CAD build for the part. Positions are in the model's coordinates, mm. Face numbers are marked on the shaded views. A direction names the side the tool comes from. Give positions to 0.01 mm unless a question says otherwise; leave off trailing zeros. Write each loop counter-clockwise with the first axis right and the second up, starting at its lowest first coordinate (ties: lowest second). Pieces come first, ordered by that corner, then holes. Notation, with made-up numbers: (36.25, 69) - (53.25, 69) arc R27 ccw to (53.25, 107) - close; hole circle Ø3 at (61.25, 64.25). An arc over 180 degrees is marked (long way). Put each result on its own line as item: value. Start each with the question number.
1. Cut at A-A on z = 270. List the corners of the cut face in (x, y).
2. Wall check: line 1 (Y direction, x = 126, z = 883); line 2 (Y direction, x = -24.5, z = 349); line 3 (X direction, y = 32, z = 335). Give the ranges that are in metal, low to high.
3. Drop flat-ended pins along their axis: pin 1 (9 mm diameter, centred on x = 5.5, y = -106.5, fed in from +Z); pin 2 (6 mm diameter, centred on x = 85, y = 5.5, fed in from -Z); pin 3 (1 mm diameter, centred on x = 45.5, z = 158, fed in from +Y). Give the stop position or say it passes through.
4. Cut at C-C on x = 117. List the corners of the cut face in (y, z), and give its area (3 significant figures).
5. Tool access for the marked faces 1, 2 and 3: list every direction of +Z, -Z, +X, -X, +Y, -Y with a clear straight run to the whole face (end or side of a thin tool).
6. Cut at B-B on x = 68.5. List the corners of the cut face in (y, z).
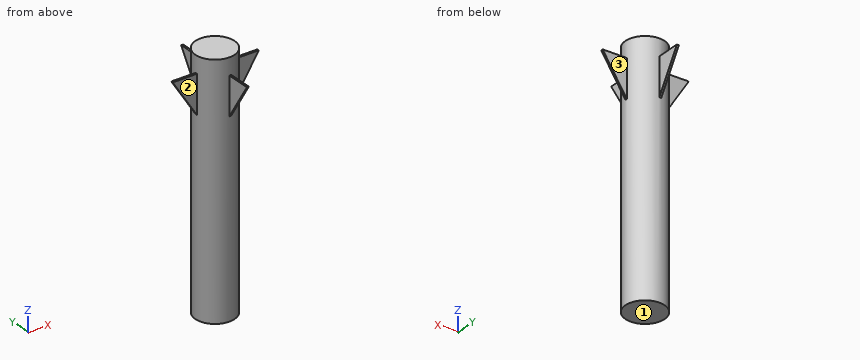
from build123d import *

# Parameters (mm, degrees)
SZKIC1_R                    = 80
DODANIE_WYCI_GNI_CIE1_DEPTH = 1000
DODANIE_WYCI_GNI_CIE2_DEPTH = 8
SZYK_KO_OWY1_COUNT          = 4


with BuildPart() as part:
    # Szkic1 → Dodanie-wyciągnięcie1 (new body)
    with BuildSketch(Plane.XY):
        Circle(SZKIC1_R)
    extrude(amount=DODANIE_WYCI_GNI_CIE1_DEPTH)

    # Szkic5 → Dodanie-wyciągnięcie2 (add)
    with BuildSketch(Plane(origin=(0, 0, 0), x_dir=(1, 0, 0), z_dir=(0, 1, 0))):
        Polygon((73.616187197, -766.737875277), (178.616187197, -931.737875277), (73.616187197, -931.737875277), align=None)
    dodanie_wyci_gni_cie2 = extrude(amount=DODANIE_WYCI_GNI_CIE2_DEPTH)

    # Szyk kołowy1: Dodanie-wyciągnięcie2 ×4 about axis
    szyk_ko_owy1_axis = Axis((0, 0, 0), (0, 0, 1))
    for i in range(1, SZYK_KO_OWY1_COUNT):
        add(dodanie_wyci_gni_cie2.rotate(szyk_ko_owy1_axis, i * 360 / SZYK_KO_OWY1_COUNT))


solid = part.part
Report:
1. outline: circle Ø160 at (0, 0)
2. line 1: y = 0 to 8
2. line 2: y = -76.16 to 76.16
2. line 3: x = -73.32 to 73.32
3. pin 1: stops at z = 931.74
3. pin 2: stops at z = 779.91
3. pin 3: stops at y = 66.14
4. outline: (0, 834.91) - (8, 834.91) - (8, 931.74) - (0, 931.74) - close
4. area: 775 mm²
5. face 1: -Z, +X, -X, +Y, -Y
5. face 2: +Z, -Z, -X, -Y
5. face 3: +Z, -Z, +X, +Y
6. outline: (-41.32, 0) - (41.32, 0) - (41.32, 1000) - (-41.32, 1000) - close
